The figure shows three views and two pictorial views of one solid part (mm, origin at its lowest corner). Answer the questions. A direction names the side the tool comes from. Coordinates: 2 decimals unless noted, no trailing zeros. Loops run counter-clockwise (first coordinate to the right, second up) from the corner with the lowest first, then second, coordinate; pieces in that order, holes last. Notation, with made-up numbers: M 25.5,2 L 55.5,2 A29 ccw 55.5,36 Z; hole C -32.75,49 d5. An arc over 180 degrees is marked long. One line per item, written item: value. Start each with the question number.
1. The part is cut by section A-A (z = 35). Write down the section's boundary in (x, y), then the cut area to 3 significant figures.
2. For the marked faces 1 and 2, determine the directions among +Z, -Z, +X, -X, +Y, -Y from which every point of the face is accessible in a straight line to the end or side of a thin tool.
3. The part is cut by section C-C (z = 20). Write down the section's boundary in (x, y), then the cut area to 3 significant figures.
4. The part is cut by section B-B (y = 24). Write down the section's boundary in (x, z), then the cut area to 3 significant figures.
5. Flat-ended cylindrical pins translate along their axes: pin 1 (6 mm diameter, centred on y = 7.5, z = 21, fed in from +X); pin 2 (2 mm diameter, centred on y = 23, z = 32.5, fed in from -X); pin 3 (2 mm diameter, centred on x = 9.5, y = 17.5, fed in from -Z); pin 4 (1 mm diameter, centred on x = 18.5, y = 23, fed in from +Z). Find the tip coordinate at first contact, or state that the pin passes through.
6. Consider probe 1 along Z at (x, y) = (3, 16); probe 2 along Y at (x, z) = (1, 35); probe 3 along X at (y, z) = (38, 28.5). Determine where each line is inside the solid, lowest interval first.
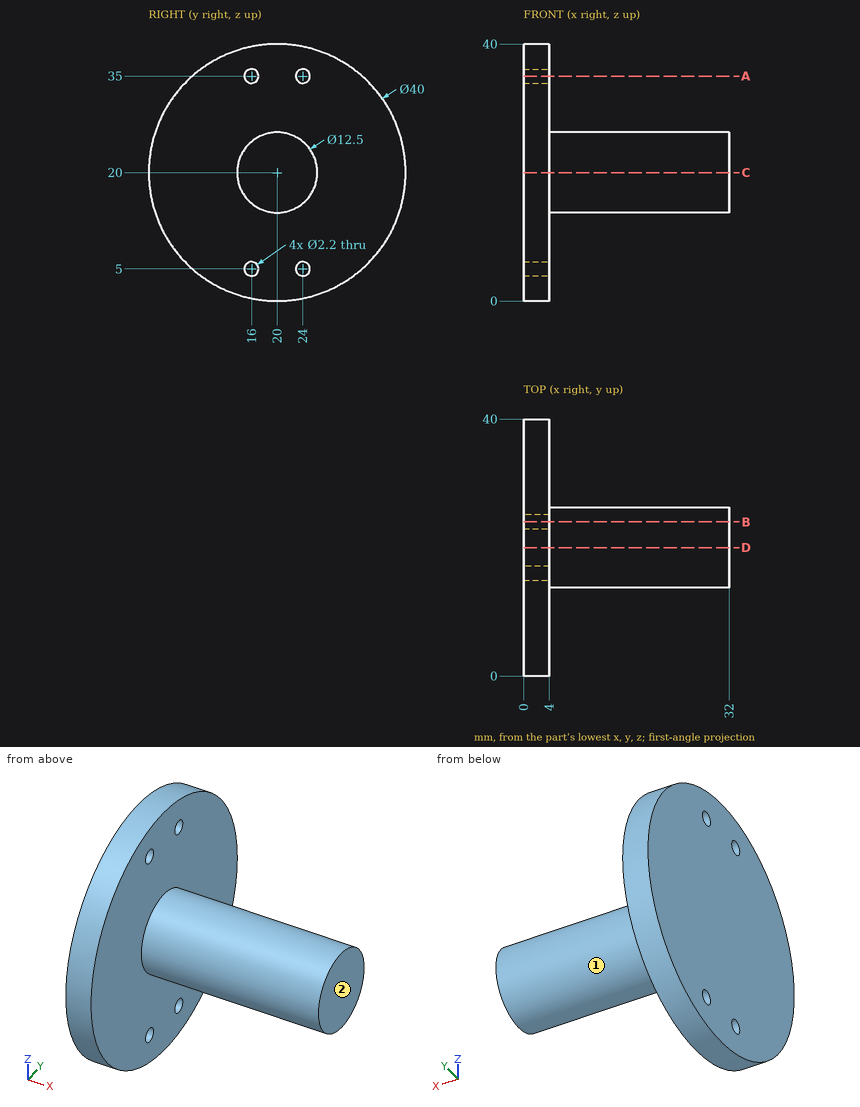
Answer block:
1. outline: M 0,6.77 L 4,6.77 L 4,14.9 L 0,14.9 Z; M 0,17.1 L 4,17.1 L 4,22.9 L 0,22.9 Z; M 0,25.1 L 4,25.1 L 4,33.23 L 0,33.23 Z
1. area: 88.2 mm2
2. face 1: +X
2. face 2: +Z, -Z, +X, +Y, -Y
3. outline: M 0,0 L 4,0 L 4,13.75 L 32,13.75 L 32,26.25 L 4,26.25 L 4,40 L 0,40 Z
3. area: 510 mm2
4. outline: M 0,0.4 L 4,0.4 L 4,3.9 L 0,3.9 Z; M 0,6.1 L 4,6.1 L 4,15.2 L 32,15.2 L 32,24.8 L 4,24.8 L 4,33.9 L 0,33.9 Z; M 0,36.1 L 4,36.1 L 4,39.6 L 0,39.6 Z
4. area: 408 mm2
5. pin 1: stops at x = 4
5. pin 2: stops at x = 0
5. pin 3: stops at z = 13.93
5. pin 4: stops at z = 25.73
6. probe 1: z = 0.4 to 3.9, 6.1 to 33.9, 36.1 to 39.6
6. probe 2: y = 6.77 to 14.9, 17.1 to 22.9, 25.1 to 33.23
6. probe 3: x = 0 to 4
